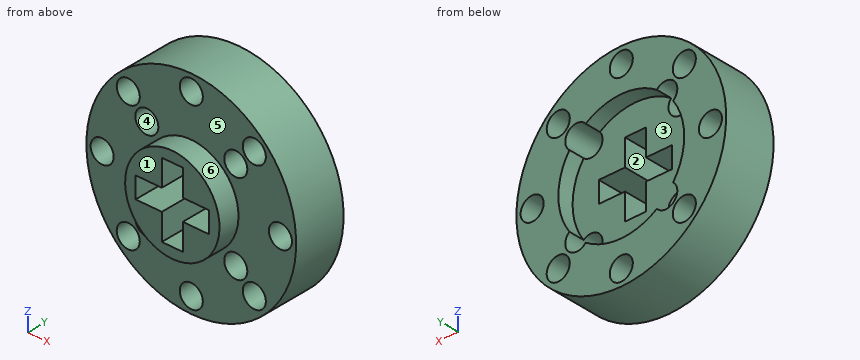
from build123d import *

# Parameters (mm, degrees)
SKETCH_1_R               = 10
EXTRUDE_1_DEPTH          = 7
SKETCH_2_R               = 1.1
CUT_EXTRUDE_1_DEPTH      = 16.779733838
PATTERN_CIRCULAR_1_COUNT = 4
PATTERN_CIRCULAR_1_ANGLE = 135
SKETCH_3_R               = 1.1
CUT_EXTRUDE_2_DEPTH      = 16.779733838
PATTERN_CIRCULAR_2_COUNT = 2
PATTERN_CIRCULAR_2_ANGLE = 90
SKETCH_4_R               = 6
CUT_EXTRUDE_3_DEPTH      = 1.5
SKETCH_5_R               = 10
SKETCH_5_R_2             = 4.5
CUT_EXTRUDE_4_DEPTH      = 2


with BuildPart() as part:
    # 草图1 → 凸台-拉伸1 (new body)
    with BuildSketch(Plane(origin=(0, 0, 0), x_dir=(1, 0, 0), z_dir=(0, 1, 0))):
        with Locations(Location((0, 0, 0), (0, 0, 270))):
            Circle(SKETCH_1_R)
        Polygon((1, 1), (3.5, 1), (3.5, -1), (1, -1), (1, -3.5), (-1, -3.5), (-1, -1), (-3.5, -1), (-3.5, 1), (-1, 1), (-1, 3.5), (1, 3.5), align=None, mode=Mode.SUBTRACT)
    extrude(amount=EXTRUDE_1_DEPTH)

    # 草图2 → 切除-拉伸1 (cut, through all)
    with BuildSketch(Plane(origin=(0, 7, 0), x_dir=(1, 0, 0), z_dir=(0, 1, 0))):
        with Locations(Location((-6.01040764, 6.01040764, 0), (0, 0, 270))):
            Circle(SKETCH_2_R)
        with Locations(Location((6.01040764, -6.01040764, 0), (0, 0, 270))):
            Circle(SKETCH_2_R)
    cut_extrude_1 = extrude(amount=-CUT_EXTRUDE_1_DEPTH, mode=Mode.SUBTRACT)

    # 阵列(圆周)1: 切除-拉伸1 ×4 about axis
    pattern_circular_1_axis = Axis((0, 0, 0), (0, -1, 0))
    for i in range(1, PATTERN_CIRCULAR_1_COUNT):
        add(cut_extrude_1.rotate(pattern_circular_1_axis, i * PATTERN_CIRCULAR_1_ANGLE / (PATTERN_CIRCULAR_1_COUNT - 1)), mode=Mode.SUBTRACT)

    # 草图3 → 切除-拉伸2 (cut, through all)
    with BuildSketch(Plane(origin=(0, 7, 0), x_dir=(1, 0, 0), z_dir=(0, 1, 0))):
        with Locations(Location((-4.242640687, 4.242640687, 0), (0, 0, 270))):
            Circle(SKETCH_3_R)
        with Locations(Location((4.242640687, -4.242640687, 0), (0, 0, 270))):
            Circle(SKETCH_3_R)
    cut_extrude_2 = extrude(amount=-CUT_EXTRUDE_2_DEPTH, mode=Mode.SUBTRACT)

    # 阵列(圆周)2: 切除-拉伸2 ×2 about axis
    pattern_circular_2_axis = Axis((0, 0, 0), (0, 1, 0))
    for i in range(1, PATTERN_CIRCULAR_2_COUNT):
        add(cut_extrude_2.rotate(pattern_circular_2_axis, i * PATTERN_CIRCULAR_2_ANGLE / (PATTERN_CIRCULAR_2_COUNT - 1)), mode=Mode.SUBTRACT)

    # 草图4 → 切除-拉伸3 (cut)
    with BuildSketch(Plane(origin=(0, 7, 0), x_dir=(1, 0, 0), z_dir=(0, 1, 0))):
        Circle(SKETCH_4_R)
    extrude(amount=-CUT_EXTRUDE_3_DEPTH, mode=Mode.SUBTRACT)

    # 草图5 → 切除-拉伸4 (cut)
    with BuildSketch(Plane.XZ):
        with Locations(Location((0, 0, 0), (0, 0, 270))):
            Circle(SKETCH_5_R)
        with Locations(Location((0, 0, 0), (0, 0, 270))):
            Circle(SKETCH_5_R_2, mode=Mode.SUBTRACT)
    extrude(amount=-CUT_EXTRUDE_4_DEPTH, mode=Mode.SUBTRACT)


solid = part.part
Design review of the part built by this model. Coordinates are the model's own, in mm. Face numbers are marked on the shaded views. A direction names the side the tool comes from. Round coordinates to 2 decimals unless told otherwise and drop trailing zeros. Loops run counter-clockwise (first coordinate to the right, second up) from the corner with the lowest first, then second, coordinate; pieces in that order, holes last. Notation, with made-up numbers: (-16.75, -35) -> (11.25, -35) arc R8 cw to (11.25, -29) -> close; hole circle Ø11 at (70, -11). An arc over 180 degrees is marked (long way). Use one line per item in the form item = value. Start each with the question number.
Q1. For pin 1 Ø3 at (x, z) = (6.01, 6.01) entering from -Y; pin 2 Ø2 at (x, y) = (2.5, 3) entering from +Z; pin 3 Ø2 at (y, z) = (2, 2) entering from -X, all flat-tipped, find the tip position at first contact; note any pin that passes through.
Q2. Wall thickness on line 1 along X through (y, z) = (4.5, 0); line 2 along Z through (x, y) = (-6.5, 4.75); line 3 along Z through (x, y) = (-5.5, 4): over which ranges is each line inside the solid? List them lowest first. Write a range as [from, to].
Q3. Machinability: for the marked faces 1, 2 and 3, which of the approach directions +Z, -Z, +X, -X, +Y, -Y give a long, thin tool a straight path to every point of the face, cutting with its end or side? Answer none if there is none.
Q4. We need section D-D on x = -3.75. Give the boundary of the cut face in (y, z), then the cut area to 3 significant figures.
Q5. Draft analysis for pull direction Z (two halves, no side actions). For the marked faces 4, 5 and 6, state which applies: +Z half, -Z half, draft (parallel to the pull), parting line (faces both ways), or undercut.
Q6. We need section B-B on y = 1. Give the boundary of the cut face in (x, z).
Q7. We need section A-A on z = 0. Give the boundary of the cut face in (x, y).
Q8. We need section C-C on z = -6.5. Give the boundary of the cut face in (x, y), then the cut area to 3 significant figures.
Calculated:
q1.pin_1 = 2
q1.pin_2 = 9.89
q1.pin_3 = -9.95
q2.line_1 = [-10, -9.6], [-7.4, -3.5], [3.5, 7.4], [9.6, 10]
q2.line_2 = [-7.6, -7], [-5.03, 5.03], [7, 7.6]
q2.line_3 = [-8.35, -6.98], [-5.04, 5.04], [6.98, 8.35]
q3.face_1 = +Z, -Z, +X, -X, -Y
q3.face_2 = +Y, -Y
q3.face_3 = +Y
q4.outline = (0, -2.49) -> (2, -2.49) -> (2, -3.26) -> (5.5, -3.26) -> (5.5, 3.26) -> (2, 3.26) -> (2, 2.49) -> (0, 2.49) -> close; (2, -9.27) -> (7, -9.27) -> (7, -5.23) -> (2, -5.23) -> close; (2, 5.23) -> (7, 5.23) -> (7, 9.27) -> (2, 9.27) -> close
q4.area = 73.2 mm²
q5.face_4 = undercut
q5.face_5 = draft
q5.face_6 = parting line
q6.outline = circle Ø9 at (0, 0); hole (-3.5, -1) -> (-1, -1) -> (-1, -3.5) -> (1, -3.5) -> (1, -1) -> (3.5, -1) -> (3.5, 1) -> (1, 1) -> (1, 3.5) -> (-1, 3.5) -> (-1, 1) -> (-3.5, 1) -> close
q7.outline = (-10, 2) -> (-9.6, 2) -> (-9.6, 7) -> (-10, 7) -> close; (-7.4, 2) -> (-4.5, 2) -> (-4.5, 0) -> (-3.5, 0) -> (-3.5, 5.5) -> (-6, 5.5) -> (-6, 7) -> (-7.4, 7) -> close; (3.5, 0) -> (4.5, 0) -> (4.5, 2) -> (7.4, 2) -> (7.4, 7) -> (6, 7) -> (6, 5.5) -> (3.5, 5.5) -> close; (9.6, 2) -> (10, 2) -> (10, 7) -> (9.6, 7) -> close
q8.outline = (-7.6, 2) -> (-7, 2) -> (-7, 7) -> (-7.6, 7) -> close; (-5.03, 2) -> (5.03, 2) -> (5.03, 7) -> (-5.03, 7) -> close; (7, 2) -> (7.6, 2) -> (7.6, 7) -> (7, 7) -> close
q8.area = 56.3 mm²
